from build123d import *

# Parameters (mm, degrees)
F0_W     = 12.7
F0_H     = 15.24
F1_DEPTH = 15.24
F2_R     = 2.38125
F3_DEPTH = 15.24
F4_W     = 12.7
F4_H     = 15.24
F5_DEPTH = 2.54
F7_R     = 1.905
F8_DEPTH = 15.241


with BuildPart() as f1:
    # F0 (on Top) → F1 (new body)
    with BuildSketch(Plane.XY):
        Rectangle(F0_W, F0_H)
    extrude(amount=F1_DEPTH)

    # F2 (on face) → F3 (join)
    with BuildSketch(Plane(origin=(0, 0, 0), x_dir=(1, 0, 0), z_dir=(0, 0, -1))):
        Circle(F2_R)
    extrude(amount=F3_DEPTH)

    # F4 (on face) → F5 (join)
    with BuildSketch(Plane.XZ.offset(7.62)):
        with Locations((12.7, 7.62)):
            Rectangle(F4_W, F4_H)
        with BuildLine():
            ThreePointArc((19.05, 0), (26.67, 7.62), (19.05, 15.24))
            Line((19.05, 15.24), (19.05, 0))
        make_face()
    extrude(amount=-F5_DEPTH)

    # F6: F1 across plane


with BuildPart() as f1_1:
    add(f1.part)
    add(f1.part.mirror(Plane.XZ))

    # F7 (on face) → F8 (cut, through all)
    with BuildSketch(Plane.XZ.offset(7.62)):
        with Locations((15.24, 7.62)):
            Circle(F7_R)
        with Locations((22.86, 7.62)):
            Circle(F7_R)
    extrude(amount=-F8_DEPTH, mode=Mode.SUBTRACT)


solid = f1_1.part
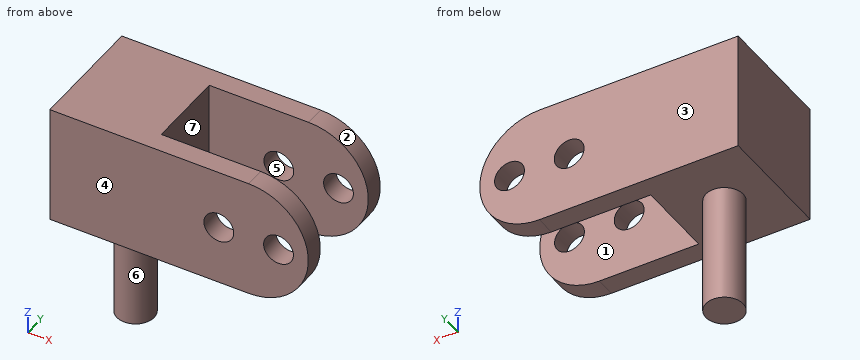
Geometry check sheet. Reference: the model listing, model coordinates, mm. Face numbers are marked on the shaded views. A direction names the side the tool comes from. Coordinates: 2 decimals unless noted, no trailing zeros. Order: outer loops, then holes, each group sorted by start corner. A loop starts at its lowest first (then second) coordinate and runs counter-clockwise, first axis right, second up. Notation, with made-up numbers: (33.25, -40) -> (59.25, -40) arc R30 cw to (59.25, -5) -> close; hole circle Ø2 at (55, -22.5). An arc over 180 degrees is marked (long way). Use a Markdown table: item, result. Add a question column.
1. Cross-section at D-D (x = 22.86). Enter the section's corners in (y, z) (3 decimals), and give its area (3 significant figures).
2. Cross-section at C-C (y = 0). Enter the section's corners in (x, z), and give its area (3 significant figures).
3. Cross-section at A-A (x = 15.24). Enter the section's corners in (y, z) (3 decimals), and give its area (3 significant figures).
4. Mould release check, pull along Y, two halves, no side actions. Record for the marked faces 1, 2, 3 and 4: pulls with the +Y half, pulls with the -Y half, needs draft (parallel to the pull), parting line crosses it, or undercut.
5. Material ranges on L1, parallel to Y at x = 17.5, z = 13.5; L2, parallel to Z at x = 15.24, y = -6 (3 decimals); L3, parallel to X at y = 1, z = 2, recorded low to high.
6. Go/stop test with flat-tipped pins: pin 1 Ø4.5 at (x, y) = (12.5, -3.5) entering from -Z; pin 2 Ø3 at (y, z) = (2, 8) entering from +X. Record where each tip stops, or that it passes through.
7. Cross-section at B-B (z = 7.62). Enter the section's corners in (x, y) (3 decimals), and give its area (3 significant figures).
8. Set-up check for the marked faces 5, 6 and 7: record each of +Z, -Z, +X, -X, +Y, -Y from which the full face is reachable in a straight line by a thin tool's end or side.
Filled sheet:
| question | item | result |
|---|---|---|
| 1 | outline | (-7.62, 1.021) -> (-5.08, 1.021) -> (-5.08, 5.715) -> (-7.62, 5.715) -> close; (-7.62, 9.525) -> (-5.08, 9.525) -> (-5.08, 14.219) -> (-7.62, 14.219) -> close; (5.08, 1.021) -> (7.62, 1.021) -> (7.62, 5.715) -> (5.08, 5.715) -> close; (5.08, 9.525) -> (7.62, 9.525) -> (7.62, 14.219) -> (5.08, 14.219) -> close |
| 1 | area | 47.7 mm2 |
| 2 | outline | (-6.35, 0) -> (-2.38, 0) -> (-2.38, -15.24) -> (2.38, -15.24) -> (2.38, 0) -> (6.35, 0) -> (6.35, 15.24) -> (-6.35, 15.24) -> close |
| 2 | area | 266 mm2 |
| 3 | outline | (-7.62, 0) -> (-5.08, 0) -> (-5.08, 5.715) -> (-7.62, 5.715) -> close; (-7.62, 9.525) -> (-5.08, 9.525) -> (-5.08, 15.24) -> (-7.62, 15.24) -> close; (5.08, 0) -> (7.62, 0) -> (7.62, 5.715) -> (5.08, 5.715) -> close; (5.08, 9.525) -> (7.62, 9.525) -> (7.62, 15.24) -> (5.08, 15.24) -> close |
| 3 | area | 58.1 mm2 |
| 4 | face 1 | undercut |
| 4 | face 2 | needs draft |
| 4 | face 3 | pulls with the +Y half |
| 4 | face 4 | pulls with the -Y half |
| 5 | L1 | -7.62 to -5.08, 5.08 to 7.62 |
| 5 | L2 | 0 to 5.715, 9.525 to 15.24 |
| 5 | L3 | -6.35 to 6.35 |
| 6 | pin 1 | z = 0 |
| 6 | pin 2 | x = 6.35 |
| 7 | outline | (-6.35, -7.62) -> (13.335, -7.62) -> (13.335, -5.08) -> (6.35, -5.08) -> (6.35, 5.08) -> (13.335, 5.08) -> (13.335, 7.62) -> (-6.35, 7.62) -> close; (17.145, -7.62) -> (20.955, -7.62) -> (20.955, -5.08) -> (17.145, -5.08) -> close; (17.145, 5.08) -> (20.955, 5.08) -> (20.955, 7.62) -> (17.145, 7.62) -> close; (24.765, -7.62) -> (26.67, -7.62) -> (26.67, -5.08) -> (24.765, -5.08) -> close; (24.765, 5.08) -> (26.67, 5.08) -> (26.67, 7.62) -> (24.765, 7.62) -> close |
| 7 | area | 258 mm2 |
| 8 | face 5 | +Y, -Y |
| 8 | face 6 | -Z |
| 8 | face 7 | +Z, -Z, +X |
